Part model, mm, in its own coordinate system. Give positions to 0.01 mm unless a question says otherwise; leave off trailing zeros. Order: outer loops, then holes, each group sorted by start corner. A loop starts at its lowest first (then second) coordinate and runs counter-clockwise, first axis right, second up. Notation, with made-up numbers: M -37,-2 L -8,-2 A23 ccw -8,30 Z; hole C -30.5,36 d8. An arc over 180 degrees is marked long. Return JSON: item names as keys, results as strings.
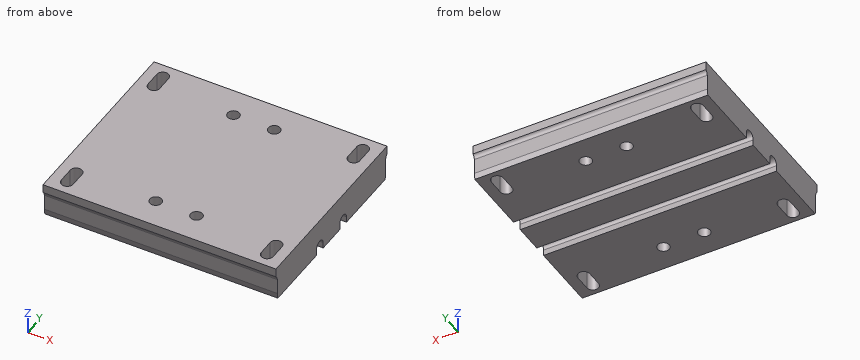
Autodesk Inventor part; units mm, degrees
ref_plane "YZ Plane" through (0, 0, 0) normal (1, 0, 0) x (0, 1, 0)
ref_plane "XZ Plane" through (0, 0, 0) normal (0, 1, 0) x (-1, 0, 0)
ref_plane "XY Plane" through (0, 0, 0) normal (0, 0, 1) x (1, 0, 0)
sketch "Sketch1" plane through (0, 0, 0) normal (0, 0, 1) x (1, 0, 0)
  circle A0 centre (10.5, 36.5) radius 3.05
  circle A1 centre (-10.5, 36.5) radius 3.05
  circle A2 centre (-10.5, -33.5) radius 3.05
  circle A3 centre (10.5, -33.5) radius 3.05
  line L0 (60, 51.5) -> (-60, 51.5)
  line L1 (-60, 51.5) -> (-60, -48.5)
  line L2 (-60, -48.5) -> (60, -48.5)
  line L3 (60, -48.5) -> (60, 51.5)
  circle A4 centre (51.5, 8.625) radius 3.05
  circle A5 centre (-51.5, -5.625) radius 3.05
  circle A6 centre (51.5, -5.625) radius 3.05
  circle A7 centre (-51.5, 8.625) radius 3.05
  arc A8 (-54.55, 36.5) -> (-48.45, 36.5) centre (-51.5, 36.5) ccw
  arc A9 (48.45, 36.5) -> (54.55, 36.5) centre (51.5, 36.5) ccw
  arc A10 (54.55, -33.5) -> (48.45, -33.5) centre (51.5, -33.5) ccw
  arc A11 (-48.45, -33.5) -> (-54.55, -33.5) centre (-51.5, -33.5) ccw
  arc A12 (-13.55, 8.625) -> (-7.45, 8.625) centre (-10.5, 8.625) ccw
  arc A13 (13.55, -5.625) -> (7.45, -5.625) centre (10.5, -5.625) ccw
  arc A14 (-7.45, -5.625) -> (-13.55, -5.625) centre (-10.5, -5.625) ccw
  arc A15 (7.45, 8.625) -> (13.55, 8.625) centre (10.5, 8.625) ccw
  line L4 (-48.45, -33.5) -> (-48.45, -41.5)
  arc A16 (-54.55, -41.5) -> (-48.45, -41.5) centre (-51.5, -41.5) ccw
  line L5 (-54.55, -41.5) -> (-54.55, -33.5)
  line L6 (54.55, -33.5) -> (54.55, -41.5)
  arc A17 (48.45, -41.5) -> (54.55, -41.5) centre (51.5, -41.5) ccw
  line L7 (48.45, -41.5) -> (48.45, -33.5)
  line L8 (-54.55, 36.5) -> (-54.55, 44.5)
  arc A18 (-48.45, 44.5) -> (-54.55, 44.5) centre (-51.5, 44.5) ccw
  line L9 (-48.45, 44.5) -> (-48.45, 36.5)
  line L10 (-7.45, -5.625) -> (-7.45, -13.625)
  arc A19 (-13.55, -13.625) -> (-7.45, -13.625) centre (-10.5, -13.625) ccw
  line L11 (-13.55, -13.625) -> (-13.55, -5.625)
  line L12 (13.55, -5.625) -> (13.55, -13.625)
  arc A20 (7.45, -13.625) -> (13.55, -13.625) centre (10.5, -13.625) ccw
  line L13 (7.45, -13.625) -> (7.45, -5.625)
  line L14 (13.55, 16.625) -> (13.55, 8.625)
  line L15 (7.45, 8.625) -> (7.45, 16.625)
  arc A21 (13.55, 16.625) -> (7.45, 16.625) centre (10.5, 16.625) ccw
  line L16 (54.55, 44.5) -> (54.55, 36.5)
  line L17 (48.45, 36.5) -> (48.45, 44.5)
  arc A22 (54.55, 44.5) -> (48.45, 44.5) centre (51.5, 44.5) ccw
  line L18 (-7.45, 16.625) -> (-7.45, 8.625)
  line L19 (-13.55, 8.625) -> (-13.55, 16.625)
  arc A23 (-7.45, 16.625) -> (-13.55, 16.625) centre (-10.5, 16.625) ccw
  point P0 (0, 0)
  point P1 (-51.375, 35)
  point P2 (51.375, 35)
  point P3 (51.375, -35)
  point P4 (-51.375, -35)
  point P5 (-10.5, 7.125)
  point P6 (10.5, -7.125)
  point P7 (-10.5, -7.125)
  point P8 (10.5, 7.125)
extrude "Extrusion1" add sketch "Sketch1" along normal blind 18 contours L3 L2 L1 L0 | A4 | A5 | A6 | A7 | L19 A23 L18 A12 | L12 A20 L13 A13 | L10 A19 L11 A14 | L15 A21 L14 A15
sketch "Sketch2" plane through (60, -48.5, 0) normal (1, 0, 0) x (0, 0, -1)
  arc A0 (-3.1, 63.55) -> (-3.1, 57.45) centre (-3.1, 60.5) ccw
  arc A1 (-3.1, 42.55) -> (-3.1, 36.45) centre (-3.1, 39.5) ccw
  line L0 (0, 0) -> (0, 100)
  line L1 (0, 100) -> (-18, 100)
  line L2 (-18, 0) -> (-18, 100)
  line L3 (0, 0) -> (-18, 0)
  circle A2 centre (66.9, 39.625) radius 3.05 construction
  circle A3 centre (66.9, 60.375) radius 3.05 construction
  circle A4 centre (-3.1, 60.375) radius 3.05 construction
  circle A5 centre (-3.1, 39.625) radius 3.05 construction
  line L4 (81.9, -10) -> (81.9, 110) construction
  line L5 (81.9, 110) -> (-18.1, 110) construction
  line L6 (-18.1, 110) -> (-18.1, -10) construction
  line L7 (-18.1, -10) -> (81.9, -10) construction
  line L8 (-3.1, -4.425) -> (0, -4.425)
  line L9 (0, -4.425) -> (0, 1.675)
  line L10 (0, 1.675) -> (-3.1, 1.675)
  line L11 (0, 100) -> (0, 0)
  line L12 (-3.1, 36.45) -> (0, 36.45)
  line L13 (0, 36.45) -> (0, 42.55)
  line L14 (0, 42.55) -> (-3.1, 42.55)
  line L15 (-3.1, 57.45) -> (0, 57.45)
  line L16 (0, 57.45) -> (0, 63.55)
  line L17 (0, 63.55) -> (-3.1, 63.55)
  line L18 (-3.1, 98.325) -> (0, 98.325)
  line L19 (0, 98.325) -> (0, 104.425)
  line L20 (0, 104.425) -> (-3.1, 104.425)
  line L21 (-3.1, -1.375) -> (-3.1, 101.375) construction
  line L22 (-3.1, 60.5) -> (-3.1, 39.5) construction
  circle A6 centre (39.025, -1.875) radius 3.05
  circle A7 centre (24.775, 101.875) radius 3.05
  circle A8 centre (24.775, -1.875) radius 3.05
  circle A9 centre (39.025, 101.875) radius 3.05
  arc A10 (66.9, 104.925) -> (66.9, 98.825) centre (66.9, 101.875) ccw
  arc A11 (66.9, 1.175) -> (66.9, -4.925) centre (66.9, -1.875) ccw
  arc A12 (-3.1, -4.925) -> (-3.1, 1.175) centre (-3.1, -1.875) ccw
  arc A13 (-3.1, 98.825) -> (-3.1, 104.925) centre (-3.1, 101.875) ccw
  arc A14 (39.025, 63.425) -> (39.025, 57.325) centre (39.025, 60.375) ccw
  arc A15 (24.775, 36.575) -> (24.775, 42.675) centre (24.775, 39.625) ccw
  arc A16 (24.775, 57.325) -> (24.775, 63.425) centre (24.775, 60.375) ccw
  arc A17 (39.025, 42.675) -> (39.025, 36.575) centre (39.025, 39.625) ccw
  line L23 (-3.1, 98.825) -> (-11.1, 98.825)
  arc A18 (-11.1, 104.925) -> (-11.1, 98.825) centre (-11.1, 101.875) ccw
  line L24 (-11.1, 104.925) -> (-3.1, 104.925)
  line L25 (-3.1, -4.925) -> (-11.1, -4.925)
  arc A19 (-11.1, 1.175) -> (-11.1, -4.925) centre (-11.1, -1.875) ccw
  line L26 (-11.1, 1.175) -> (-3.1, 1.175)
  line L27 (66.9, 104.925) -> (74.9, 104.925)
  arc A20 (74.9, 98.825) -> (74.9, 104.925) centre (74.9, 101.875) ccw
  line L28 (74.9, 98.825) -> (66.9, 98.825)
  line L29 (24.775, 57.325) -> (16.775, 57.325)
  arc A21 (16.775, 63.425) -> (16.775, 57.325) centre (16.775, 60.375) ccw
  line L30 (16.775, 63.425) -> (24.775, 63.425)
  line L31 (24.775, 36.575) -> (16.775, 36.575)
  arc A22 (16.775, 42.675) -> (16.775, 36.575) centre (16.775, 39.625) ccw
  line L32 (16.775, 42.675) -> (24.775, 42.675)
  line L33 (47.025, 36.575) -> (39.025, 36.575)
  line L34 (39.025, 42.675) -> (47.025, 42.675)
  arc A23 (47.025, 36.575) -> (47.025, 42.675) centre (47.025, 39.625) ccw
  line L35 (74.9, -4.925) -> (66.9, -4.925)
  line L36 (66.9, 1.175) -> (74.9, 1.175)
  arc A24 (74.9, -4.925) -> (74.9, 1.175) centre (74.9, -1.875) ccw
  line L37 (47.025, 57.325) -> (39.025, 57.325)
  line L38 (39.025, 63.425) -> (47.025, 63.425)
  arc A25 (47.025, 57.325) -> (47.025, 63.425) centre (47.025, 60.375) ccw
  point P0 (0, 48.5)
  point P1 (-3.1, 50)
  point P2 (-18, 50)
  point P3 (-3.1, 50)
  point P4 (-3.1, 50)
  point P5 (-3.1, 50)
  point P6 (-3.1, 50)
  point P7 (66.9, 101.375)
  point P8 (66.9, -1.375)
  point P9 (-3.1, -1.375)
  point P10 (-3.1, 101.375)
  point P11 (39.025, 60.5)
  point P12 (24.775, 39.5)
  point P13 (24.775, 60.5)
  point P14 (39.025, 39.5)
  dimension "d2" = 6.1
  dimension "d3" = 3.1
  dimension "d4" = 21
  dimension "d5" = 102.75
  dimension "d6" = 6.1
  dimension "d7" = 6.1
  dimension "d8" = 6.1
sketch "Sketch2 outline for Extrusion2" plane through (60, -48.5, 0) normal (1, 0, 0) x (0, 0, -1)
  line L0 (-11.1, -4.925) -> (-3.1, -4.925)
  arc A0 (-11.1, 1.175) -> (-11.1, -4.925) centre (-11.1, -1.875) ccw
  line L1 (-3.1, 1.175) -> (-11.1, 1.175)
  line L2 (0, 1.675) -> (-3.1, 1.175)
  line L3 (0, -4.425) -> (0, 1.675)
  line L4 (-3.1, -4.925) -> (0, -4.425)
  line L5 (0, 104.425) -> (0, 98.325)
  line L6 (0, 98.325) -> (-3.1, 98.825)
  line L7 (-3.1, 98.825) -> (-11.1, 98.825)
  arc A1 (-11.1, 98.825) -> (-11.1, 104.925) centre (-11.1, 101.875) cw
  line L8 (-11.1, 104.925) -> (-3.1, 104.925)
  line L9 (-3.1, 104.925) -> (0, 104.425)
  line L10 (0, 36.45) -> (0, 42.55)
  line L11 (-3.1, 36.45) -> (0, 36.45)
  arc A2 (-3.1, 42.55) -> (-3.1, 36.45) centre (-3.1, 39.5) ccw
  line L12 (0, 42.55) -> (-3.1, 42.55)
  line L13 (0, 57.45) -> (0, 63.55)
  line L14 (-3.1, 57.45) -> (0, 57.45)
  arc A3 (-3.1, 63.55) -> (-3.1, 57.45) centre (-3.1, 60.5) ccw
  line L15 (0, 63.55) -> (-3.1, 63.55)
extrude "Extrusion2" cut sketch "Sketch2 outline for Extrusion2" against normal through all
properties part number "AXYZ" material "PC/ABS Plastic"
Q1. Band-saw the part on B-B (x = 51.5). Give the cut face in (y, z) (3 decimals).
Established:
{"outline": "M -48.5,13.506 A3.05 cw -47.325,11.1 L -47.325,3.1 L -46.825,0 L -44.55,0 L -44.55,18 L -48.5,18 Z; M -30.45,0 L -12.05,0 L -12.05,3.1 A3.05 cw -5.95,3.1 L -5.95,0 L 8.95,0 L 8.95,3.1 A3.05 cw 15.05,3.1 L 15.05,0 L 33.45,0 L 33.45,18 L -30.45,18 Z; M 47.55,0 L 49.825,0 L 50.325,3.1 L 50.325,11.1 A3.05 cw 51.5,13.506 L 51.5,18 L 47.55,18 Z"}
Q2. Probe line 1 along Y through (x, z) = (10.5, 13.5); line 2 along Y through (x, z) = (10.5, 10.25) (3 decimals); line 3 along Y through (x, z) = (-10.5, 4.5) (3 decimals). List the from-to ranges inside material, lowest first.
Established:
{"line 1": "y = -48.49 to -36.55, -30.45 to 33.45, 39.55 to 51.49", "line 2": "y = -47.325 to -36.55, -30.45 to 33.45, 39.55 to 50.325", "line 3": "y = -47.325 to -36.55, -30.45 to -11.71, -6.29 to 9.29, 14.71 to 33.45, 39.55 to 50.325"}
Q3. Pin check, flat tips, straight feed: pin 1 (0.9 mm diameter, centred on x = -2.5, z = 1, fed in from -Y); pin 2 (1.6 mm diameter, centred on x = 16.5, z = 1, fed in from +Y); pin 3 (3.5 mm diameter, centred on x = -15.5, z = 1.5, fed in from -Y) (3 decimals). Stop position of each tip, or through.
Established:
{"pin 1": "stops at y = -47.06", "pin 2": "stops at y = 50.12", "pin 3": "stops at y = -47.325"}
Q4. Band-saw the part on A-A (z = 15.75). Give the number of separate pieces and of enclosed holes in the cut face, then the cut area to 3 significant figures.
Established:
{"separate pieces": "1", "enclosed holes": "8", "area": "11,600 mm²"}
Q5. Band-saw the part on D-D (x = 2). Give the cut face in (y, z) (3 decimals), then the cut area to 3 significant figures.
Established:
{"outline": "M -48.5,13.506 A3.05 cw -47.325,11.1 L -47.325,3.1 L -46.825,0 L -12.05,0 L -12.05,3.1 A3.05 cw -5.95,3.1 L -5.95,0 L 8.95,0 L 8.95,3.1 A3.05 cw 15.05,3.1 L 15.05,0 L 49.825,0 L 50.325,3.1 L 50.325,11.1 A3.05 cw 51.5,13.506 L 51.5,18 L -48.5,18 Z", "area": "1,700 mm²"}
